Read the model definition and answer for the solid it produces. Units are mm, in the model's axes. A direction names the side the tool comes from. Round coordinates to 2 decimals unless told otherwise and drop trailing zeros. Order: outer loops, then holes, each group sorted by start corner. A loop starts at its lowest first (then second) coordinate and runs counter-clockwise, first axis right, second up. Notation, with made-up numbers: (10.25, -39) - (47.25, -39) arc R16 cw to (47.25, -31) - close; hole circle Ø10 at (-15, 76.5). An arc over 180 degrees is marked (long way). Answer as a JSON object with one key per item and string values. Group by question number.
Q1. Consider line 1 (X direction, y = 0, z = -9.25); line 2 (Y direction, x = 0.75, z = -6.5); line 3 (X direction, y = -0.5, z = -12.25). Determine where each line is inside the solid, lowest interval first.
Q2. A tool of negligible diameter and unlimited length cuts with its end or side. For faces 4 (the flat face through (-2, 0, -13.5)), 5 (the cylindrical face through (-1.952, -0.434, -0.254)), 6 (the conical face through (0.644, 2.043, -6.814)), from which of +Z, -Z, +X, -X, +Y, -Y can it reach the whole face along a straight path? Write none if from no direction.
Q3. A cutting plane is placed at A-A on y = 0. Determine the outline of the cut face in (x, z).
Q4. A cutting plane is placed at C-C on x = 2.75. Determine the outline of the cut face in (y, z), and give its area (3 significant figures).
Q5. Given pin 1 Ø2 at (x, z) = (-0.5, -11.5) entering from -Y; pin 2 Ø3 at (y, z) = (-1, -9.5) entering from +X; pin 3 Ø1.5 at (y, z) = (-1.5, -11) entering from +X; pin 4 Ø3 at (x, z) = (-0.5, -5.5) entering from -Y, each flat-ended and moving along its own axis, determine where each tip first touches the part or whether it passes through.
Q6. The mould has two halves that part along X. Classify faces 1 (the cylindrical face through (-2.44, -0.54, -10.15)), 2 (the cylindrical face through (0.07, -1.5, -6.66)), 3 (the flat face through (-2, -2, -12)): pulls with the +X half, pulls with the -X half, needs draft (parallel to the pull), parting line crosses it, or undercut.
```python
from build123d import *


with BuildPart() as part:
    # Sketch1 → Revolve1 (revolve)
    with BuildSketch(Plane(origin=(0, 0, 0), x_dir=(0, 0, -1), z_dir=(1, 0, 0))):
        with BuildLine():
            Line((6.244562647, 2), (8.244562647, 2.5))
            Line((8.244562647, 2.5), (12, 2.5))
            Line((12, 2.5), (12, 3.5))
            Line((12, 3.5), (13.5, 3.5))
            Line((13.5, 3.5), (13.5, 1.5))
            Line((13.5, 1.5), (0, 1.5))
            Line((0, 1.5), (0, 2))
            Line((0, 2), (0.5, 2))
            ThreePointArc((0.5, 2), (3.372281323, 3.5), (6.244562647, 2))
        make_face()
    revolve(axis=Axis((0, 0, 0), (0, 0, -1)))


solid = part.part
```
Result set:
{
 "1": {"line 1": "x = -2.5 to -1.5, 1.5 to 2.5", "line 2": "y = -1.92 to -1.3, 1.3 to 1.92", "line 3": "x = -3.46 to -1.41, 1.41 to 3.46"},
 "2": {"face 4": "-Z, +X, -X, +Y, -Y", "face 5": "+Z", "face 6": "none"},
 "3": {"outline": "(-3.5, -13.5) - (-1.5, -13.5) - (-1.5, 0) - (-2, 0) - (-2, -0.5) arc R3.5 ccw to (-2, -6.24) - (-2.5, -8.24) - (-2.5, -12) - (-3.5, -12) - close; (1.5, -13.5) - (3.5, -13.5) - (3.5, -12) - (2.5, -12) - (2.5, -8.24) - (2, -6.24) arc R3.5 ccw to (2, -0.5) - (2, 0) - (1.5, 0) - close"},
 "4": {"outline": "(-2.17, -13.5) - (2.17, -13.5) - (2.17, -12) - (-2.17, -12) - close; circle Ø4.33 at (0, -3.37)", "area": "21.2 mm²"},
 "5": {"pin 1": "stops at y = -3.5", "pin 2": "stops at x = 2.5", "pin 3": "stops at x = 2.38", "pin 4": "stops at y = -3.43"},
 "6": {"face 1": "parting line crosses it", "face 2": "undercut", "face 3": "needs draft"}
}
